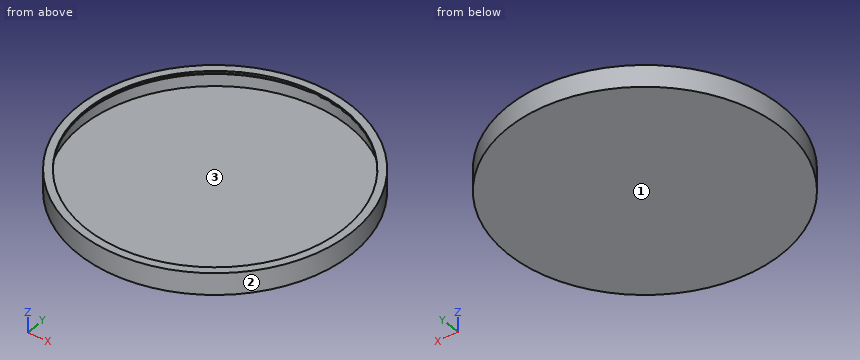
from build123d import *

# Parameters (mm, degrees)
SKETCH006_R     = 44
PAD002_DEPTH    = 7
SKETCH007_R     = 41.5
POCKET004_DEPTH = 6
SKETCH008_R     = 43
POCKET005_DEPTH = 4.5
FILLET002_R     = 1


with BuildPart() as part:
    # Sketch006 → Pad002 (new body)
    with BuildSketch(Plane.XY):
        Circle(SKETCH006_R)
    extrude(amount=PAD002_DEPTH)

    # Sketch007 (on Face3 of Pad002) → Pocket004 (cut)
    with BuildSketch(Plane.XY.offset(7)):
        Circle(SKETCH007_R)
    extrude(amount=-POCKET004_DEPTH, mode=Mode.SUBTRACT)

    # Sketch008 → Pocket005 (cut)
    with BuildSketch(Plane.XY.offset(1)):
        Circle(SKETCH008_R)
    extrude(amount=POCKET005_DEPTH, mode=Mode.SUBTRACT)

    # Fillet002
    fillet002_edges = [part.edges().sort_by_distance(p)[0] for p in [
        (-41.5, 0, 5.5),
    ]]
    fillet(fillet002_edges, radius=FILLET002_R)


solid = part.part
Work out the finished part from the listing and answer in its coordinate system (mm). Face numbers are marked on the shaded views. Give positions to 0.01 mm unless a question says otherwise; leave off trailing zeros. Order: outer loops, then holes, each group sorted by start corner. A loop starts at its lowest first (then second) coordinate and runs counter-clockwise, first axis right, second up. Notation, with made-up numbers: M 61.5,63 L 93.5,63 A7 cw 93.5,74 Z; hole C 36,-17.75 d8. An arc over 180 degrees is marked long. Return JSON: item names as keys, results as strings.
Q1. The mould has two halves that part along X. Classify the marked faces 1, 2 and 3: pulls with the +X half, pulls with the -X half, needs draft (parallel to the pull), parting line crosses it, or undercut.
Answer below:
{"face 1": "needs draft", "face 2": "parting line crosses it", "face 3": "undercut"}
Q2. Find section B-B, the plane y = 0. Write down the section's boundary in (x, z), and give its area (3 significant figures).
Answer below:
{"outline": "M -44,0 L 44,0 L 44,7 L 41.5,7 L 41.5,6.5 A1 ccw 42.5,5.5 L 43,5.5 L 43,1 L -43,1 L -43,5.5 L -42.5,5.5 A1 ccw -41.5,6.5 L -41.5,7 L -44,7 Z", "area": "104 mm^2"}
Q3. Find section A-A, the plane z = 3.5. Write down the section's boundary in (x, y), and give its area (3 significant figures).
Answer below:
{"outline": "C 0,0 d88; hole C 0,0 d86", "area": "273 mm^2"}
Q4. Find the intervals of material crossed by line 1 along Y through (x, z) = (0, 6.8); line 2 along Y through (x, z) = (0, 3.4); line 3 along Z through (x, y) = (-32.5, 0), in increasing order. Write a range as [from, to].
Answer below:
{"line 1": "y = [-44, -41.5], [41.5, 44]", "line 2": "y = [-44, -43], [43, 44]", "line 3": "z = [0, 1]"}
Q5. Each of these flat-tipped pins is pushed along its axis until it touches: pin 1 (4 mm diameter, centred on x = 18.5, z = 3, fed in from +Y); pin 2 (3 mm diameter, centred on x = -18, z = 2.5, fed in from -Y); pin 3 (2 mm diameter, centred on x = -30, z = 6, fed in from -Y). Where does it stop, or does it pass through?
Answer below:
{"pin 1": "stops at y = 40.79", "pin 2": "stops at y = -40.79", "pin 3": "stops at y = -33.09"}
